Source: CAD feature listing. Evaluate the final solid. Frame: model axes, mm. A direction names the side the tool comes from. Round coordinates to 2 decimals unless told otherwise and drop trailing zeros. Loops run counter-clockwise (first coordinate to the right, second up) from the corner with the lowest first, then second, coordinate; pieces in that order, holes last. Notation, with made-up numbers: M 68.5,47.25 L 120.5,47.25 A17 ccw 120.5,56.25 Z; hole C -39,-31 d2. An arc over 180 degrees is marked long. Answer as a JSON object with one key per item and string values.
from build123d import *

# Parameters (mm, degrees)
SKETCH_1_W             = 40
SKETCH_1_H             = 18
EXTRUDE_1_DEPTH        = 10
CUT_EXTRUDE_1_DEPTH    = 3
CUT_EXTRUDE_2_DEPTH    = 1.5
CHAMFER_1_SIZE         = 1
CHAMFER_2_SIZE         = 1
CHAMFER_2_SIZE2        = 1.732050808
CHAMFER_2_PART_2_SIZE  = 1
CHAMFER_2_PART_2_SIZE2 = 1.732050808
FILLET_1_R             = 1


with BuildPart() as part:
    # 草图1 → 凸台-拉伸1 (new body)
    with BuildSketch(Plane(origin=(0, 0, 0), x_dir=(1, 0, 0), z_dir=(0, 1, 0))):
        with Locations((20, 9)):
            Rectangle(SKETCH_1_W, SKETCH_1_H)
        with BuildLine():
            Line((17, 5.7), (8, 5.7))
            ThreePointArc((8, 5.7), (4.7, 9), (8, 12.3))
            Line((8, 12.3), (17, 12.3))
            ThreePointArc((17, 12.3), (20.3, 9), (17, 5.7))
        make_face(mode=Mode.SUBTRACT)
    extrude(amount=EXTRUDE_1_DEPTH)

    # 草图2 → 切除-拉伸1 (cut)
    with BuildSketch(Plane.XZ):
        with BuildLine():
            Line((40, -5.7), (40, -12.3))
            Line((40, -12.3), (8, -12.3))
            ThreePointArc((8, -12.3), (4.7, -9), (8, -5.7))
            Line((8, -5.7), (40, -5.7))
        make_face()
    extrude(amount=-CUT_EXTRUDE_1_DEPTH, mode=Mode.SUBTRACT)

    # 草图3 → 切除-拉伸2 (cut)
    with BuildSketch(Plane.XZ):
        Polygon((0, -5.7), (4.7, -5.7), (4.7, 0), (11.3, 0), (11.3, -18), (4.7, -18), (4.7, -12.3), (0, -12.3), align=None)
    extrude(amount=-CUT_EXTRUDE_2_DEPTH, mode=Mode.SUBTRACT)

    # 倒角1
    chamfer_1_edges = [part.edges().sort_by_distance(p)[0] for p in [
        (0, 0, -15.15),
        (0, 0, -2.85),
        (4.7, 0, -2.85),
        (4.7, 0, -15.15),
    ]]
    chamfer(chamfer_1_edges, length=CHAMFER_1_SIZE)

    # 倒角2
    chamfer_2_edges = [part.edges().sort_by_distance(p)[0] for p in [
        (11.3, 0, -2.85),
    ]]
    chamfer_2_side = [part.faces().sort_by_distance(p)[0] for p in [
        (11.3, 0.75, -2.85),
    ]]
    chamfer(chamfer_2_edges, length=CHAMFER_2_SIZE, length2=CHAMFER_2_SIZE2, reference=chamfer_2_side[0])

    # 倒角2 part 2
    chamfer_2_part_2_edges = [part.edges().sort_by_distance(p)[0] for p in [
        (11.3, 0, -15.15),
    ]]
    chamfer_2_part_2_side = [part.faces().sort_by_distance(p)[0] for p in [
        (11.3, 0.75, -15.15),
    ]]
    chamfer(chamfer_2_part_2_edges, length=CHAMFER_2_PART_2_SIZE, length2=CHAMFER_2_PART_2_SIZE2, reference=chamfer_2_part_2_side[0])

    # 圆角1
    fillet_1_edges = [part.edges().sort_by_distance(p)[0] for p in [
        (20, 10, -18),
        (40, 10, -9),
        (20, 10, 0),
        (0, 10, -9),
        (40, 5, 0),
        (40, 5, -18),
        (0, 5.5, -18),
        (0, 5.5, 0),
        (40, 0, -15.15),
        (40, 0, -2.85),
    ]]
    fillet(fillet_1_edges, radius=FILLET_1_R)


solid = part.part
Item 1: Section C-C on x = 36. Return the cut outline in (y, z), then the cut area to 3 significant figures.
Answer sheet:
{"outline": "M 0,-18 L 9,-18 A1 ccw 10,-17 L 10,-1 A1 ccw 9,0 L 0,0 L 0,-5.7 L 3,-5.7 L 3,-12.3 L 0,-12.3 Z", "area": "160 mm²"}
Item 2: Section B-B on z = -9. Return the cut outline in (x, y), then the cut area to 3 significant figures.
Answer sheet:
{"outline": "M 0,1.5 L 4.7,1.5 L 4.7,10 L 1,10 A1 ccw 0,9 Z; M 20.3,3 L 40,3 L 40,9 A1 ccw 39,10 L 20.3,10 Z", "area": "177 mm²"}
Item 3: Line query: probe 1 along X at (y, z) = (1.25, -15); probe 2 along Y at (x, z) = (23.5, -7); probe 3 along Y at (x, z) = (11, -13.25). Output: solid intervals per line, ascending. Write a range as from..to.
Answer sheet:
{"probe 1": "x = 0..4.7, 11.3..40", "probe 2": "y = 3..10", "probe 3": "y = 1.5..10"}
Item 4: Contact query for flat-ended pins moving along their axis: pin 1 Ø3 at (x, z) = (34, -7) entering from -Y; pin 2 Ø5.5 at (x, z) = (8.5, -13) entering from -Y; pin 3 Ø3.5 at (x, z) = (23.5, -9) entering from -Y; pin 4 Ø6 at (x, z) = (9.5, -2) entering from -Y. Output: stop coordinate, or through.
Answer sheet:
{"pin 1": "stops at y = 0", "pin 2": "stops at y = 1.5", "pin 3": "stops at y = 3", "pin 4": "stops at y = 0.31"}
Item 5: Access query for faces 5 (the flat face through (4, 1.5, -9)), 6 (the flat face through (20, 4, 0)), 7 (the flat face through (2, 1, -12.3)), 8 (the flat face through (4.2, 0.5, -2.9)), 9 (the cylindrical face through (20.3, 6.5, -9.1)). Directions: +Z, -Z, +X, -X, +Y, -Y. A direction counts if a zero-diameter tool reaches every point of the face in a straight line with its end or side. Return the directions, or none.
Answer sheet:
{"face 5": "-Y", "face 6": "+Z, +X, -X, +Y, -Y", "face 7": "+X, -X, -Y", "face 8": "+Z, -Z, -Y", "face 9": "+Y, -Y"}
Item 6: Section D-D on y = 2. Return the cut outline in (x, z).
Answer sheet:
{"outline": "M 0,-17 A1 ccw 1,-18 L 39,-18 A1 ccw 40,-17 L 40,-12.3 L 8,-12.3 A3.3 cw 8,-5.7 L 40,-5.7 L 40,-1 A1 ccw 39,0 L 1,0 A1 ccw 0,-1 Z"}
Item 7: Pull-direction query (X, two-part tool) for faces 1 (the flat face through (12.18, 0.49, -15.11)), 2 (the cylindrical face through (39.699, 0.285, -15.19)), 3 (the flat face through (0.5, 0.5, -15.1)), 4 (the cylindrical face through (20.266, 9.715, -0.301)); classes: pulls with the +X half, pulls with the -X half, needs draft (parallel to the pull), parting line crosses it, or undercut.
Answer sheet:
{"face 1": "undercut", "face 2": "pulls with the +X half", "face 3": "pulls with the -X half", "face 4": "needs draft"}
Item 8: Section A-A on y = 8. Return the cut outline in (x, z), then the cut area to 3 significant figures.
Answer sheet:
{"outline": "M 0,-17 A1 ccw 1,-18 L 39,-18 A1 ccw 40,-17 L 40,-1 A1 ccw 39,0 L 1,0 A1 ccw 0,-1 Z; hole M 8,-12.3 L 17,-12.3 A3.3 ccw 17,-5.7 L 8,-5.7 A3.3 ccw Z", "area": "626 mm²"}
